Work out the finished part from the listing and answer in its coordinate system (mm). A direction names the side the tool comes from. Give positions to 0.01 mm unless a question says otherwise; leave off trailing zeros. Loops run counter-clockwise (first coordinate to the right, second up) from the corner with the lowest first, then second, coordinate; pieces in that order, holes last.
from build123d import *

# Parameters (mm, degrees)
F0_W     = 97.1741192043
F0_H     = 70.9515530616
F1_DEPTH = 25
F2_R     = 15
F3_SIZE  = 5
F4_R     = 5
F5_T     = -2.5
F6_R     = 1


with BuildPart() as f1:
    # F0 (on Top) → F1 (new body)
    with BuildSketch(Plane.XY):
        with Locations((-16.4708662778, 12.1098598465)):
            Rectangle(F0_W, F0_H)
    extrude(amount=F1_DEPTH)

    # F2
    f2_edges = [f1.edges().sort_by_distance(p)[0] for p in [
        (-65.057926, -23.365917, 12.5),
        (32.116193, -23.365917, 12.5),
        (32.116193, 47.585636, 12.5),
        (-65.057926, 47.585636, 12.5),
    ]]
    fillet(f2_edges, radius=F2_R)

    # F3
    f3_edges = [f1.edges().sort_by_distance(p)[0] for p in [
        (-65.057926, 12.10986, 25),
    ]]
    chamfer(f3_edges, length=F3_SIZE)

    # F4
    f4_edges = [f1.edges().sort_by_distance(p)[0] for p in [
        (-65.057926, 12.10986, 20),
        (-60.057926, 12.10986, 25),
    ]]
    fillet(f4_edges, radius=F4_R)

    # F5
    f5_openings = [f1.faces().sort_by_distance(p)[0] for p in [
        (-16.470866, 12.10986, 0),
    ]]
    offset(amount=F5_T, openings=f5_openings)

    # F6
    f6_edges = [f1.edges().sort_by_distance(p)[0] for p in [
        (-16.470866, -20.865917, 0),
        (-60.664528, -18.972518, 0),
    ]]
    fillet(f6_edges, radius=F6_R)


solid = f1.part
Item 1: For faces 5 (the face through (25.548, -16.614, 23.205)), 6 (the face through (29.616, 12, 9)), determine the directions among +Z, -Z, +X, -X, +Y, -Y from which every point of the face is accessible in a straight line to the end or side of a thin tool.
Item 2: Determine the mould class of faces 1 (the face through (25.364, 41.017, 23.205)), 2 (the face through (-17, -20.866, 9)), 3 (the face through (-59.926, 12.397, 24.609)), 4 (the face through (24.289, 39.918, 21.207)) for opening direction Y: released by +Y, released by -Y, zero draft, split by the parting line, or undercut.
Item 3: Find section A-A, the plane z = 5.5. Write down the section's boundary in (x, y).
Item 4: Find section B-B, the plane x = -38. Write down the section's boundary in (y, z).
Item 5: Find section C-C, the plane y = -3. Write down the section's boundary in (x, z).
Item 6: Flat-ended cylindrical pins translate along their axes: pin 1 Ø3 at (x, y) = (1.5, 30.5) entering from -Z; pin 2 Ø12 at (x, y) = (-44.5, -14.5) entering from -Z; pin 3 Ø1 at (y, z) = (5.5, 22) entering from -X. Find the tip coordinate at first contact, or state that the pin passes through.
Item 7: Consider line 1 (Y direction, x = -19, z = 3.5); line 2 (X direction, y = -7.5, z = 5); line 3 (Z direction, x = 3.5, y = 30). Determine where each line is inside the solid, lowest interval first.
Ans:
1. face 5: +Z, +X, -Y
1. face 6: -Z
2. face 1: released by +Y
2. face 2: undercut
2. face 3: zero draft
2. face 4: undercut
3. outline: (-65.06, -8.37) arc R15 ccw to (-50.06, -23.37) - (17.12, -23.37) arc R15 ccw to (32.12, -8.37) - (32.12, 32.59) arc R15 ccw to (17.12, 47.59) - (-50.06, 47.59) arc R15 ccw to (-65.06, 32.59) - close; hole (-62.56, -8.37) arc R12.5 ccw to (-50.06, -20.87) - (17.12, -20.87) arc R12.5 ccw to (29.62, -8.37) - (29.62, 32.59) arc R12.5 ccw to (17.12, 45.09) - (-50.06, 45.09) arc R12.5 ccw to (-62.56, 32.59) - close
4. outline: (-23.37, 1) arc R1 ccw to (-22.37, 0) - (-21.87, 0) arc R1 ccw to (-20.87, 1) - (-20.87, 17.93) arc R2.5 cw to (-20.13, 19.7) - (-18.06, 21.77) arc R2.5 cw to (-16.29, 22.5) - (40.51, 22.5) arc R2.5 cw to (42.28, 21.77) - (44.35, 19.7) arc R2.5 cw to (45.09, 17.93) - (45.09, 1) arc R1 ccw to (46.09, 0) - (46.59, 0) arc R1 ccw to (47.59, 1) - (47.59, 17.93) arc R5 ccw to (46.12, 21.46) - (44.05, 23.54) arc R5 ccw to (40.51, 25) - (-16.29, 25) arc R5 ccw to (-19.83, 23.54) - (-21.9, 21.46) arc R5 ccw to (-23.37, 17.93) - close
5. outline: (-65.06, 1) arc R1 ccw to (-64.06, 0) - (-63.56, 0) arc R1 ccw to (-62.56, 1) - (-62.56, 17.93) arc R2.5 cw to (-61.83, 19.7) - (-59.75, 21.77) arc R2.5 cw to (-57.99, 22.5) - (25.05, 22.5) arc R2.5 cw to (26.81, 21.77) - (28.88, 19.7) arc R2.5 cw to (29.62, 17.93) - (29.62, 1) arc R1 ccw to (30.62, 0) - (31.12, 0) arc R1 ccw to (32.12, 1) - (32.12, 17.93) arc R5 ccw to (30.65, 21.46) - (28.58, 23.54) arc R5 ccw to (25.05, 25) - (-57.99, 25) arc R5 ccw to (-61.52, 23.54) - (-63.59, 21.46) arc R5 ccw to (-65.06, 17.93) - close
6. pin 1: stops at z = 22.5
6. pin 2: stops at z = 19.23
6. pin 3: stops at x = -63.56
7. line 1: y = -23.37 to -20.87, 45.09 to 47.59
7. line 2: x = -65.06 to -62.56, 29.62 to 32.12
7. line 3: z = 22.5 to 25
